CAD build for the part. Positions are in the model's coordinates, mm. Face numbers are marked on the shaded views. A direction names the side the tool comes from. Round coordinates to 2 decimals unless told otherwise and drop trailing zeros. Loops run counter-clockwise (first coordinate to the right, second up) from the corner with the lowest first, then second, coordinate; pieces in that order, holes last. Notation, with made-up numbers: (-30.75, -3.5) - (9.25, -3.5) arc R15 ccw to (9.25, 1.5) - close; hole circle Ø10 at (89, -14.5). An arc over 180 degrees is marked (long way). One line per question, with ' | ' between items.
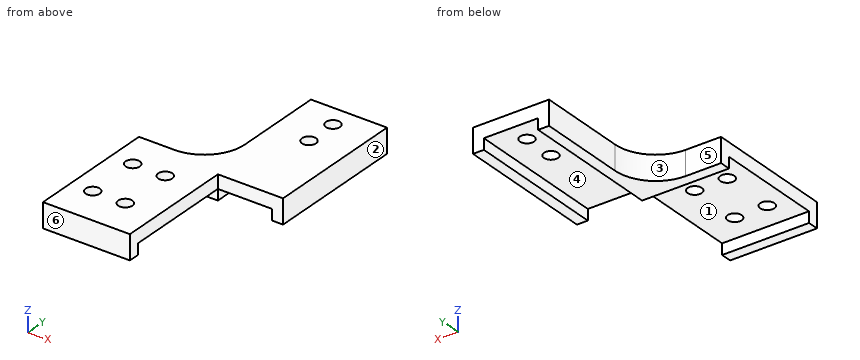
```python
from build123d import *

# Parameters (mm, degrees)
SKETCH1_R           = 2.6
BOSS_EXTRUDE1_DEPTH = 5
SKETCH3_W           = 32
SKETCH3_H           = 4
SKETCH3_W_2         = 4
SKETCH3_H_2         = 52
BOSS_EXTRUDE3_DEPTH = 4
FILLET1_R           = 15


with BuildPart() as part:
    # Sketch1 → Boss-Extrude1 (new body)
    with BuildSketch(Plane.XY):
        Polygon((-11.163233534, 11.489286615), (-39.163233534, 11.489286615), (-39.163233534, -36.510713385), (-7.163233534, -36.510713385), (-7.163233534, 7.489286615), (16.836766466, 7.489286615), (16.836766466, 59.489286615), (-11.163233534, 59.489286615), align=None)
        with Locations((-31.163233534, -22.510713385)):
            Circle(SKETCH1_R, mode=Mode.SUBTRACT)
        with Locations((-19.163233534, -22.510713385)):
            Circle(SKETCH1_R, mode=Mode.SUBTRACT)
        with Locations((-31.163233534, -2.510713385)):
            Circle(SKETCH1_R, mode=Mode.SUBTRACT)
        with Locations((-19.163233534, -2.510713385)):
            Circle(SKETCH1_R, mode=Mode.SUBTRACT)
        with Locations((2.836766466, 39.489286615)):
            Circle(SKETCH1_R, mode=Mode.SUBTRACT)
        with Locations((2.836766466, 51.489286615)):
            Circle(SKETCH1_R, mode=Mode.SUBTRACT)
    extrude(amount=BOSS_EXTRUDE1_DEPTH)

    # Sketch3 → Boss-Extrude3 (add)
    with BuildSketch(Plane(origin=(0, 0, 0), x_dir=(-1, 0, 0), z_dir=(0, 0, -1))):
        with Locations((23.163233534, -34.510713385)):
            Rectangle(SKETCH3_W, SKETCH3_H)
        Polygon((39.163233534, 11.489286615), (11.163233534, 11.489286615), (11.163233534, 59.489286615), (7.163233534, 59.489286615), (7.163233534, 7.489286615), (39.163233534, 7.489286615), align=None)
        with Locations((-14.836766466, 33.489286615)):
            Rectangle(SKETCH3_W_2, SKETCH3_H_2)
    extrude(amount=BOSS_EXTRUDE3_DEPTH)

    # Fillet1
    fillet1_edges = [part.edges().sort_by_distance(p)[0] for p in [
        (-11.163233534, 11.489286615, 0.5),
    ]]
    fillet(fillet1_edges, radius=FILLET1_R)


solid = part.part
```
(1) Tool access for the marked faces 5 and 6: list every direction of +Z, -Z, +X, -X, +Y, -Y with a clear straight run to the whole face (end or side of a thin tool).
Results found:
face 5: +Z, -Z, -X, +Y | face 6: +Z, -Z, +X, -X, -Y
(2) Drop flat-ended pins along their axis: P1, Ø2.5, axis at y = -22, z = 1.5, coming from the +X side; P2, Ø1.5, axis at x = -16, z = 2.5, coming from the +Y side; P3, Ø10, axis at x = -8.5, y = -17.5, coming from the -Z side. Give the stop position or say it passes through.
Results found:
P1: stops at x = -7.16 | P2: stops at y = 16.2 | P3: stops at z = 0
(3) Two-plate mould, pull along X, no slides. Class the marked faces 1, 2, 3 and 4: released by +X, released by -X, zero draft, split by the parting line, or undercut.
Results found:
face 1: zero draft | face 2: released by +X | face 3: released by -X | face 4: undercut
(4) Probe L1, parallel to X at y = 30, z = -2.5; L2, parallel to Y at x = -32, z = 4; L3, parallel to Y at x = -35.5, z = 2.25. List the from-to ranges inside material, lowest first.
Results found:
L1: x = -11.16 to -7.16, 12.84 to 16.84 | L2: y = -36.51 to -24.97, -20.05 to -4.97, -0.05 to 11.49 | L3: y = -36.51 to 11.49
(5) Cut at D-D, the plane z = 4. Write the cut outline in (x, y), then the cut area to 3 significant figures.
Results found:
outline: (-39.16, -36.51) - (-7.16, -36.51) - (-7.16, 7.49) - (16.84, 7.49) - (16.84, 59.49) - (-11.16, 59.49) - (-11.16, 26.49) arc R15 cw to (-26.16, 11.49) - (-39.16, 11.49) - close; hole circle Ø5.2 at (-31.16, -22.51); hole circle Ø5.2 at (-31.16, -2.51); hole circle Ø5.2 at (-19.16, -22.51); hole circle Ø5.2 at (-19.16, -2.51); hole circle Ø5.2 at (2.84, 39.49); hole circle Ø5.2 at (2.84, 51.49) | area: 2,900 mm²
(6) Cut at C-C, the plane x = 4. Write the cut outline in (y, z), then the cut area to 3 significant figures.
Results found:
outline: (7.49, 0) - (37.16, 0) - (37.16, 5) - (7.49, 5) - close; (41.81, 0) - (49.16, 0) - (49.16, 5) - (41.81, 5) - close; (53.81, 0) - (59.49, 0) - (59.49, 5) - (53.81, 5) - close | area: 213 mm²
(7) Cut at B-B, the plane y = 27.5. Write the cut outline in (x, z), then the cut area to 3 significant figures.
Results found:
outline: (-11.16, -4) - (-7.16, -4) - (-7.16, 0) - (12.84, 0) - (12.84, -4) - (16.84, -4) - (16.84, 5) - (-11.16, 5) - close | area: 172 mm²
(8) Cut at A-A, the plane z = -1.5. Write the cut outline in (x, y).
Results found:
outline: (-39.16, -36.51) - (-7.16, -36.51) - (-7.16, -32.51) - (-39.16, -32.51) - close; (-39.16, 7.49) - (-7.16, 7.49) - (-7.16, 59.49) - (-11.16, 59.49) - (-11.16, 26.49) arc R15 cw to (-26.16, 11.49) - (-39.16, 11.49) - close; (12.84, 7.49) - (16.84, 7.49) - (16.84, 59.49) - (12.84, 59.49) - close
